```python
from build123d import *

# Parameters (mm, degrees)
SKETCH1_R           = 6.25
SKETCH1_R_2         = 9.5
BOSS_EXTRUDE1_DEPTH = 10
SKETCH4_R           = 6.25
BOSS_EXTRUDE3_DEPTH = 8


with BuildPart() as part:
    # Sketch1 → Boss-Extrude1 (new body)
    with BuildSketch(Plane(origin=(0, 0, 0), x_dir=(1, 0, 0), z_dir=(0, 1, 0))):
        with BuildLine():
            Line((-37.5, 0), (-37.5, -300))
            Line((-37.5, -300), (37.5, -300))
            Line((37.5, -300), (37.5, 0))
            ThreePointArc((37.5, 0), (0, 37.5), (-37.5, 0))
        make_face()
        with Locations(Location((0, -150, 0), (0, 0, 270))):
            Circle(SKETCH1_R, mode=Mode.SUBTRACT)
        with Locations(Location((0, 0, 0), (0, 0, 270))):
            Circle(SKETCH1_R_2, mode=Mode.SUBTRACT)
    extrude(amount=BOSS_EXTRUDE1_DEPTH)

    # Sketch4 → Boss-Extrude3 (add)
    with BuildSketch(Plane(origin=(37.5, 0, 0), x_dir=(0, 0, -1), z_dir=(1, 0, 0))):
        with BuildLine():
            Line((-240, 0), (-240, 10))
            Line((-240, 10), (-273.641101056, 37.717797887))
            ThreePointArc((-273.641101056, 37.717797887), (-276.621981266, 39.412172408), (-280, 40))
            Line((-280, 40), (-290, 40))
            ThreePointArc((-290, 40), (-297.071067812, 37.071067812), (-300, 30))
            Line((-300, 30), (-300, 0))
            Line((-300, 0), (-240, 0))
        make_face()
        with Locations((-285, 25)):
            Circle(SKETCH4_R, mode=Mode.SUBTRACT)
    boss_extrude3 = extrude(amount=BOSS_EXTRUDE3_DEPTH)

    # Mirror1: Boss-Extrude3 across plane
    add(boss_extrude3.mirror(Plane(origin=(0, 0, 0), x_dir=(0, 0, 1), z_dir=(1, 0, 0))))


solid = part.part
```
Work out the finished part from the listing and answer in its coordinate system (mm). A direction names the side the tool comes from. Coordinates: 2 decimals unless noted, no trailing zeros. Write each loop counter-clockwise with the first axis right and the second up, starting at its lowest first coordinate (ties: lowest second). Pieces come first, ordered by that corner, then holes.
Q1. Which of the six approach directions +Z, -Z, +X, -X, +Y, -Y give full straight-line access (tool end or side, diameter ignored) to faces 5 (the face through (-41, 5, 240)), 6 (the face through (37.5, 5, 122)), 7 (the face through (0.82, 4.93, -37.49)), 8 (the face through (37.5, 22, 277))?
Q2. Determine the mould class of faces 1 (the face through (-45.5, 16, 277)), 2 (the face through (1, 0, 134)), 3 (the face through (-41.444, 25.275, 291.244)), 4 (the face through (41.444, 25.275, 291.244)) for opening direction Y: released by +Y, released by -Y, zero draft, split by the parting line, or undercut.
Q3. A cutting plane is placed at D-D, the plane y = 15.5. Give the vertices of the cut face in (x, z), then the cut area to 3 significant figures.
Q4. Find the intervals of material crossed by line 1 (Y direction, x = -40, z = 285); line 2 (X direction, y = 2, z = 150); line 3 (Y direction, x = -3.5, z = 172), in increasing order.
Q5. Each of these flat-tipped pins is pushed along its axis until it touches: pin 1 Ø5 at (x, z) = (-12, 161.5) entering from +Y; pin 2 Ø3 at (y, z) = (3, 144.5) entering from -X; pin 3 Ø7.5 at (y, z) = (25, 285) entering from +X; pin 4 Ø8 at (x, y) = (-36.5, 21) entering from -Z. Where does it stop, or does it pass through?
Q6. A cutting plane is placed at A-A, the plane x = 0. Give the vertices of the cut face in (y, z), then the cut area to 3 significant figures.
Q7. A cutting plane is placed at C-C, the plane z = 285. Give the vertices of the cut face in (x, y), then the cut area to 3 significant figures.
Q8. A cutting plane is placed at B-B, the plane z = 150. Give the vertices of the cut face in (x, y).
Findings below:
1. face 5: -Z, -X, +Y, -Y
1. face 6: -Z, +X, +Y, -Y
1. face 7: -Z, +Y, -Y
1. face 8: +Z, -Z, +Y
2. face 1: zero draft
2. face 2: released by -Y
2. face 3: undercut
2. face 4: undercut
3. outline: (-45.5, 246.68) - (-37.5, 246.68) - (-37.5, 300) - (-45.5, 300) - close; (37.5, 246.68) - (45.5, 246.68) - (45.5, 300) - (37.5, 300) - close
3. area: 853 mm2
4. line 1: y = 0 to 18.75, 31.25 to 40
4. line 2: x = -37.5 to -6.25, 6.25 to 37.5
4. line 3: y = 0 to 10
5. pin 1: stops at y = 10
5. pin 2: stops at x = -37.5
5. pin 3: passes through
5. pin 4: stops at z = 248.65
6. outline: (0, -37.5) - (10, -37.5) - (10, -9.5) - (0, -9.5) - close; (0, 9.5) - (10, 9.5) - (10, 143.75) - (0, 143.75) - close; (0, 156.25) - (10, 156.25) - (10, 300) - (0, 300) - close
6. area: 3,060 mm2
7. outline: (-45.5, 0) - (45.5, 0) - (45.5, 18.75) - (37.5, 18.75) - (37.5, 10) - (-37.5, 10) - (-37.5, 18.75) - (-45.5, 18.75) - close; (-45.5, 31.25) - (-37.5, 31.25) - (-37.5, 40) - (-45.5, 40) - close; (37.5, 31.25) - (45.5, 31.25) - (45.5, 40) - (37.5, 40) - close
7. area: 1,190 mm2
8. outline: (-37.5, 0) - (-6.25, 0) - (-6.25, 10) - (-37.5, 10) - close; (6.25, 0) - (37.5, 0) - (37.5, 10) - (6.25, 10) - close
